from build123d import *

# Parameters (mm, degrees)
SKETCH3_W           = 210
SKETCH3_H           = 150
BOSS_EXTRUDE3_DEPTH = 3
CUT_EXTRUDE2_DEPTH  = 10
SKETCH6_R           = 6.123115527
SKETCH6_R_2         = 6.021528495
CUT_EXTRUDE4_DEPTH  = 10


with BuildPart() as part:
    # Sketch3 → Boss-Extrude3 (new body)
    with BuildSketch(Plane.XY):
        with Locations((56.698645522, -91.038012074)):
            Rectangle(SKETCH3_W, SKETCH3_H)
    extrude(amount=-BOSS_EXTRUDE3_DEPTH)

    # Sketch4 → Cut-Extrude2 (cut)
    with BuildSketch(Plane.XY):
        Polygon((35.083968717, -90.087026863), (-4.916031283, -89.786592431), (-4.916031283, -124.598736124), (35.083968717, -124.598736124), align=None)
        Polygon((-4.916031283, -84.565090297), (-4.916031283, -89.786592431), (35.083968717, -90.087026863), (35.083968717, -84.565090297), align=None)
    extrude(amount=-CUT_EXTRUDE2_DEPTH, mode=Mode.SUBTRACT)

    # Sketch6 → Cut-Extrude4 (cut)
    with BuildSketch(Plane.XY):
        with Locations((-13.502002571, -45.038518666)):
            Circle(SKETCH6_R)
        with Locations((-13.502002571, -29.469595459)):
            Circle(SKETCH6_R_2)
    extrude(amount=-CUT_EXTRUDE4_DEPTH, mode=Mode.SUBTRACT)


solid = part.part
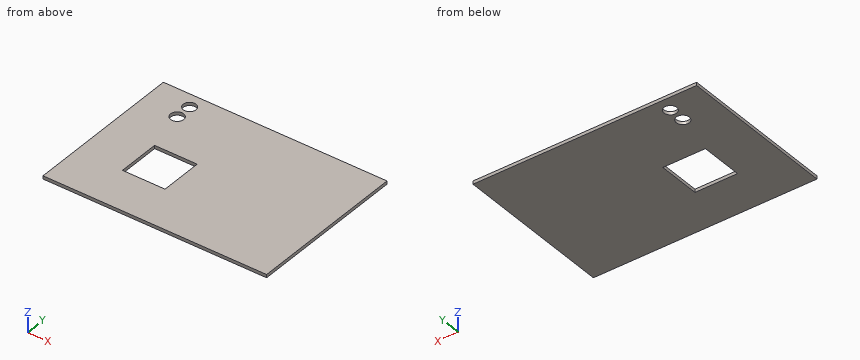
Can you work these out from the model? Positions are in its coordinate system, mm. Round coordinates to 2 decimals unless told otherwise and drop trailing zeros. Loops run counter-clockwise (first coordinate to the right, second up) from the corner with the lowest first, then second, coordinate; pieces in that order, holes last. Notation, with made-up numbers: (56, 73) - (60, 73) arc R30 ccw to (60, 110) - close; hole circle Ø11 at (15.25, -25). An arc over 180 degrees is marked (long way). Use CSV: the item, a comma, the result in double quotes. Start each with the question number.
1) If we section it at A-A on x = 32: Write out the boundary of the cut face in (y, z).
2) Please list where these lines run through material, in increasing order: probe 1 along Y at (x, z) = (7.5, -1.35); probe 2 along X at (y, z) = (-95, -1.1). Write a range as [from, to].
3) If we section it at B-B on y = -90.5: Write out the boundary of the cut face in (x, z).
4) If we section it at C-C on z = -2.5: Write out the boundary of the cut face in (x, y), plus the area to 3 significant figures.
5) For pin 1 Ø3 at (x, y) = (1, -125) entering from +Z, with a flat end and sliding along its axis, tell me the tip position at first contact or that it passes through.
Geometry results:
1,outline,"(-166.04, -3) - (-124.6, -3) - (-124.6, 0) - (-166.04, 0) - close; (-84.57, -3) - (-16.04, -3) - (-16.04, 0) - (-84.57, 0) - close"
2,probe 1,"y = [-166.04, -124.6], [-84.57, -16.04]"
2,probe 2,"x = [-48.3, -4.92], [35.08, 161.7]"
3,outline,"(-48.3, -3) - (-4.92, -3) - (-4.92, 0) - (-48.3, 0) - close; (35.08, -3) - (161.7, -3) - (161.7, 0) - (35.08, 0) - close"
4,outline,"(-48.3, -166.04) - (161.7, -166.04) - (161.7, -16.04) - (-48.3, -16.04) - close; hole circle Ø12.25 at (-13.5, -45.04); hole circle Ø12.04 at (-13.5, -29.47); hole (-4.92, -124.6) - (35.08, -124.6) - (35.08, -84.57) - (-4.92, -84.57) - close"
4,area,"29,700 mm2"
5,pin 1,"stops at z = 0"
